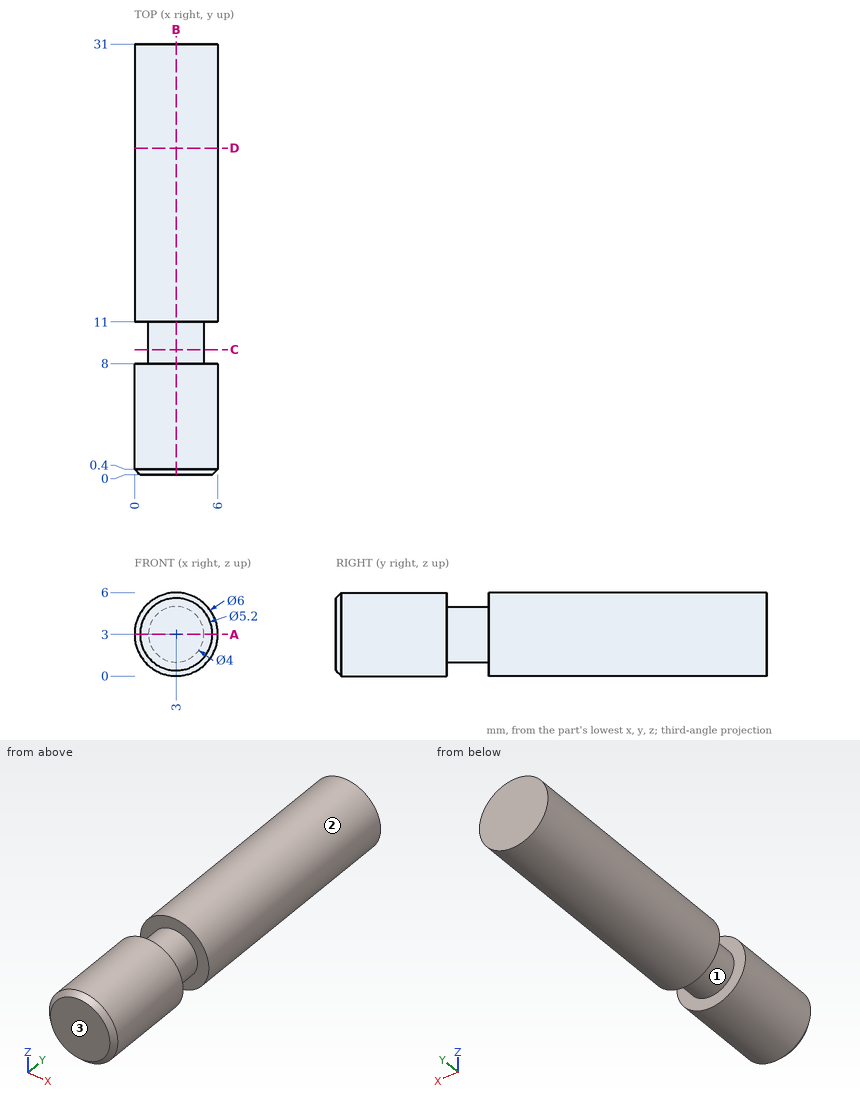
Input: dimensioned drawing with shaded views. Units: mm. Origin: part minimum x, y, z. Give positions to 0.01 mm unless a question says otherwise; leave off trailing zeros. Order: outer loops, then holes, each group sorted by start corner. A loop starts at its lowest first (then second) coordinate and runs counter-clockwise, first axis right, second up. Notation, with made-up numbers: (63, 18.5) -> (81, 18.5) arc R23 cw to (81, 45.5) -> close; hole circle Ø3 at (-25, 52.25). An arc over 180 degrees is marked (long way). Use one line per item in the form item = value.
1) Section A-A, the plane z = 3. Return loops of the section in (x, y).
Response values:
outline = (0, 0.4) -> (0.4, 0) -> (5.6, 0) -> (6, 0.4) -> (6, 8) -> (5, 8) -> (5, 11) -> (6, 11) -> (6, 31) -> (0, 31) -> (0, 11) -> (1, 11) -> (1, 8) -> (0, 8) -> close
2) Mould query, pull axis Y, two halves, no side actions, for the marked faces 1, 2 and 3. Classes: pulls with the +Y half, pulls with the -Y half, needs draft (parallel to the pull), parting line crosses it, or undercut.
Response values:
face_1 = undercut
face_2 = needs draft
face_3 = pulls with the -Y half
3) Section C-C, the plane y = 9. Return loops of the section in (x, z), and give its area (3 significant figures).
Response values:
outline = circle Ø4 at (3, 3)
area = 12.6 mm^2
4) Line query: probe 1 along Y at (x, z) = (3.25, 5.1); probe 2 along Y at (x, z) = (5.65, 3.45); probe 3 along X at (y, z) = (16.5, 1.5). Output: solid intervals per line, ascending.
Response values:
probe_1 = 0 to 8, 11 to 31
probe_2 = 0.09 to 8, 11 to 31
probe_3 = 0.4 to 5.6
5) Section B-B, the plane x = 3. Return loops of the section in (y, z).
Response values:
outline = (0, 0.4) -> (0.4, 0) -> (8, 0) -> (8, 1) -> (11, 1) -> (11, 0) -> (31, 0) -> (31, 6) -> (11, 6) -> (11, 5) -> (8, 5) -> (8, 6) -> (0.4, 6) -> (0, 5.6) -> close
6) Section D-D, the plane y = 23.5. Return loops of the section in (x, z).
Response values:
outline = circle Ø6 at (3, 3)
